Input: dimensioned drawing with shaded views. Units: mm. Origin: part minimum x, y, z. Round coordinates to 2 decimals unless told otherwise and drop trailing zeros. Loops run counter-clockwise (first coordinate to the right, second up) from the corner with the lowest first, then second, coordinate; pieces in that order, holes last. Notation, with made-up numbers: (-19.5, 21.5) - (-9.5, 21.5) arc R20 cw to (-9.5, 46.5) - close; hole circle Ø4 at (11, 81). An arc over 180 degrees is marked (long way). Answer as CSV lines item,"result".
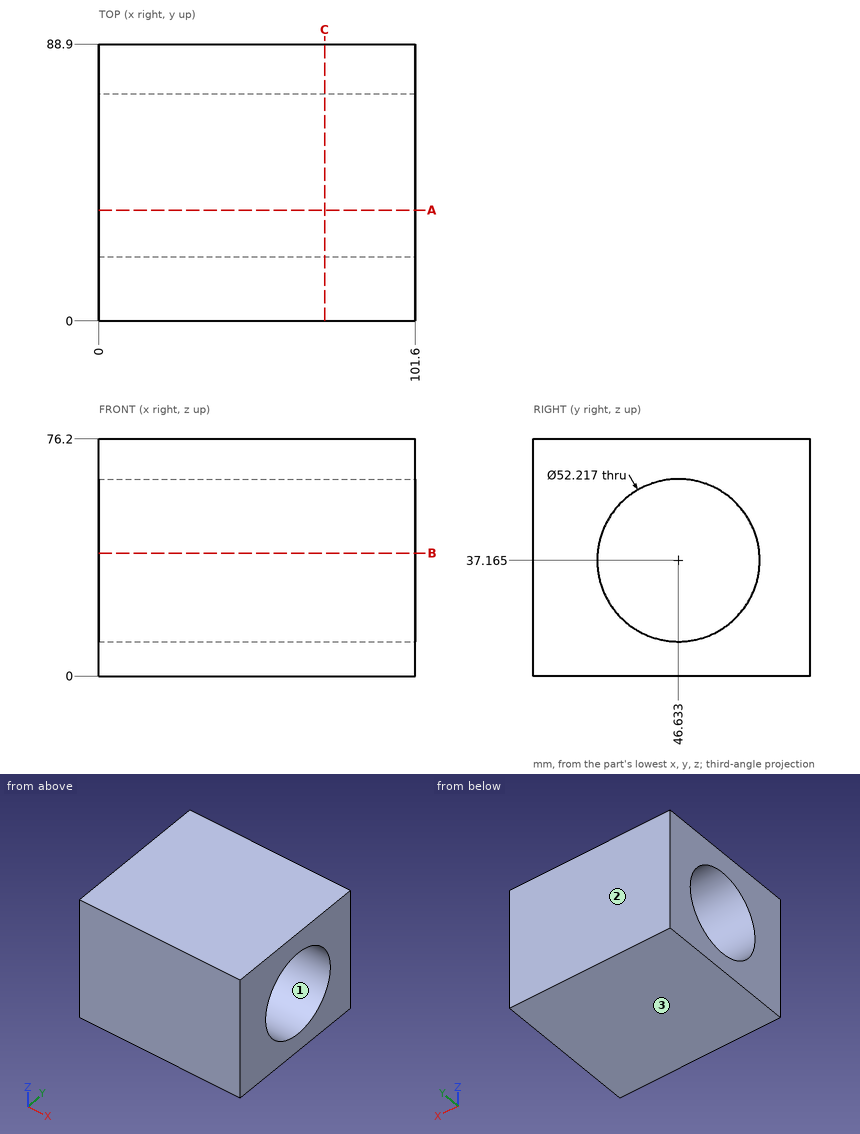
(1) Draft query along Z for the marked faces 1, 2 and 3. Return one class per face: pulls with the +Z half, pulls with the -Z half, needs draft (parallel to the pull), parting line crosses it, or undercut.
Findings below:
face 1,"undercut"
face 2,"needs draft"
face 3,"pulls with the -Z half"
(2) Section B-B (z = 39.5). Output: boundary loops of the cut face in (x, y).
Findings below:
outline,"(0, 0) - (101.6, 0) - (101.6, 20.63) - (0, 20.63) - close; (0, 72.64) - (101.6, 72.64) - (101.6, 88.9) - (0, 88.9) - close"
(3) Pin query (flat end, axial travel): P1, Ø12, axis at y = 26.5, z = 63, coming from the -X side; P2, Ø1, axis at y = 52.5, z = 62, coming from the -X side. Return the tip coordinate at first contact, or that it passes through.
Findings below:
P1,"x = 0"
P2,"through"
(4) Section A-A (y = 35.5). Output: boundary loops of the cut face in (x, z).
Findings below:
outline,"(0, 0) - (101.6, 0) - (101.6, 13.55) - (0, 13.55) - close; (0, 60.78) - (101.6, 60.78) - (101.6, 76.2) - (0, 76.2) - close"
(5) Material intervals for line 1 along Y through (x, z) = (59, 37.5); line 2 along Z through (x, y) = (11, 64.5) (1 decimal); line 3 along Y through (x, z) = (13.5, 19.5) (1 decimal), sorted ascending.
Findings below:
line 1,"0 to 20.53, 72.74 to 88.9"
line 2,"0 to 18.1, 56.2 to 76.2"
line 3,"0 to 27.4, 65.9 to 88.9"
(6) Section C-C (x = 72.5). Output: boundary loops of the cut face in (y, z) (1 decimal), and give its area (3 significant figures).
Findings below:
outline,"(0, 0) - (88.9, 0) - (88.9, 76.2) - (0, 76.2) - close; hole circle Ø52.2 at (46.6, 37.2)"
area,"4,630 mm2"
